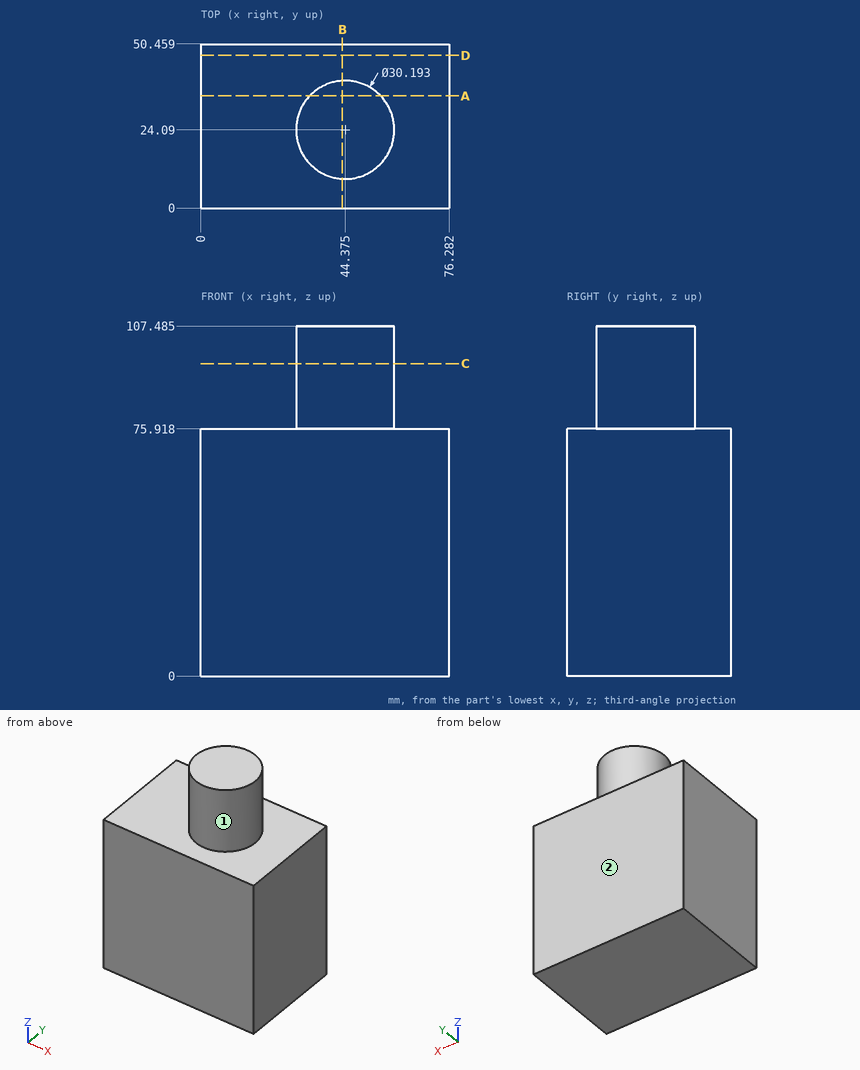
Study the drawing (mm; zero at the part's minimum x, y, z) and answer. A direction names the side the tool comes from. Round coordinates to 2 decimals unless told otherwise and drop trailing zeros. Order: outer loops, then holes, each group sorted by start corner. A loop starts at its lowest first (then second) coordinate and runs counter-clockwise, first axis right, second up. Notation, with made-up numbers: M 21,21.25 L 59,21.25 A6 cw 59,28.25 Z; hole C 30,42.25 d4. An arc over 180 degrees is marked long. One line per item, written item: value.
Q1. Find section A-A on y = 34.5. Write down the section's boundary in (x, z) (1 decimal), then the cut area to 3 significant figures.
Derived:
outline: M 0,0 L 76.3,0 L 76.3,75.9 L 55.3,75.9 L 55.3,107.5 L 33.4,107.5 L 33.4,75.9 L 0,75.9 Z
area: 6,480 mm²
Q2. Find section D-D on y = 47. Write down the section's boundary in (x, z).
Derived:
outline: M 0,0 L 76.28,0 L 76.28,75.92 L 0,75.92 Z
Q3. Find section C-C on z = 96. Write down the section's boundary in (x, y) (1 decimal).
Derived:
outline: C 44.4,24.1 d30.2
Q4. Flat-ended cylindrical pins translate along their axes: pin 1 (10 mm diameter, centred on x = 28, z = 92.5, fed in from -Y) (1 decimal); pin 2 (3 mm diameter, centred on x = 24, y = 32.5, fed in from +Z); pin 3 (5 mm diameter, centred on y = 26.5, z = 80.5, fed in from +X). Find the tip coordinate at first contact, or state that the pin passes through.
Derived:
pin 1: y = 14.2
pin 2: z = 75.92
pin 3: x = 59.47
Q5. Straight lines are drawn through the part: line 1 (Z direction, x = 39.5, y = 43.5); line 2 (Y direction, x = 47, z = 94); line 3 (X direction, y = 20, z = 102). For each, find the intervals that lie inside material, in ascending order.
Derived:
line 1: 0 to 75.92
line 2: 9.22 to 38.96
line 3: 29.84 to 58.91
Q6. Find section B-B on x = 43.5. Write down the section's boundary in (y, z) (1 decimal).
Derived:
outline: M 0,0 L 50.5,0 L 50.5,75.9 L 39.2,75.9 L 39.2,107.5 L 9,107.5 L 9,75.9 L 0,75.9 Z
Q7. For the marked faces 1 and 2, determine the directions among +Z, -Z, +X, -X, +Y, -Y from which every point of the face is accessible in a straight line to the end or side of a thin tool.
Derived:
face 1: +Z
face 2: +Z, -Z, +X, -X, +Y
